from build123d import *

# Parameters (mm, degrees)
SKETCH1_W                                       = 67
SKETCH1_H                                       = 24
BOSS_EXTRUDE1_DEPTH                             = 3.175
CSK_FOR_M2_FLAT_HEAD_MACHINE_SCREW1_D           = 2.2
CSK_FOR_M2_FLAT_HEAD_MACHINE_SCREW1_CSINK_D     = 4.4
CSK_FOR_M2_FLAT_HEAD_MACHINE_SCREW1_CSINK_ANGLE = 90
CHAMFER1_SIZE                                   = 2
CHAMFER1_SIZE2                                  = 2.383507185
SKETCH4_W                                       = 55
SKETCH4_H                                       = 10
CUT_EXTRUDE1_DEPTH                              = 36.725769761
FILLET2_R                                       = 2
FILLET4_R                                       = 3
FILLET5_R                                       = 2


with BuildPart() as part:
    # Sketch1 → Boss-Extrude1 (new body)
    with BuildSketch(Plane(origin=(0, 0, 0), x_dir=(1, 0, 0), z_dir=(0, 1, 0))):
        Rectangle(SKETCH1_W, SKETCH1_H)
    extrude(amount=BOSS_EXTRUDE1_DEPTH)

    # CSK for M2 Flat Head Machine Screw1 (through all)
    with Locations(Plane(origin=(0, 3.175, 0), x_dir=(1, 0, 0), z_dir=(0, 1, 0))):
        with Locations((-30.7, 8.5), (-30.7, -2.5), (30.7, -2.5), (30.7, 8.5)):
            CounterSinkHole(CSK_FOR_M2_FLAT_HEAD_MACHINE_SCREW1_D / 2, CSK_FOR_M2_FLAT_HEAD_MACHINE_SCREW1_CSINK_D / 2, counter_sink_angle=CSK_FOR_M2_FLAT_HEAD_MACHINE_SCREW1_CSINK_ANGLE)

    # Chamfer1
    chamfer1_edges = [part.edges().sort_by_distance(p)[0] for p in [
        (0, 0, 12),
    ]]
    chamfer1_side = [part.faces().sort_by_distance(p)[0] for p in [
        (0, 1.5875, 12),
    ]]
    chamfer(chamfer1_edges, length=CHAMFER1_SIZE, length2=CHAMFER1_SIZE2, reference=chamfer1_side[0])

    # Sketch4 → Cut-Extrude1 (cut, through all)
    with BuildSketch(Plane(origin=(0, 3.175, 0), x_dir=(1, 0, 0), z_dir=(0, 1, 0))):
        with Locations((0, 12)):
            Rectangle(SKETCH4_W, SKETCH4_H)
    extrude(amount=-CUT_EXTRUDE1_DEPTH, mode=Mode.SUBTRACT)

    # Fillet2
    fillet2_edges = [part.edges().sort_by_distance(p)[0] for p in [
        (0, 0, 9.616492815),
    ]]
    fillet(fillet2_edges, radius=FILLET2_R)

    # Fillet4
    fillet4_edges = [part.edges().sort_by_distance(p)[0] for p in [
        (-27.5, 1.5875, -7),
        (27.5, 1.5875, -7),
    ]]
    fillet(fillet4_edges, radius=FILLET4_R)

    # Fillet5
    fillet5_edges = [part.edges().sort_by_distance(p)[0] for p in [
        (33.5, 1.5875, -12),
        (33.5, 2.5875, 12),
        (-33.5, 2.5875, 12),
        (-27.5, 1.5875, -12),
        (27.5, 1.5875, -12),
        (-33.5, 1.5875, -12),
    ]]
    fillet(fillet5_edges, radius=FILLET5_R - 0.0001)  # a hair under: the kernel refuses the full size


solid = part.part
Could you check a few things on this model? Use its own coordinates, in mm. A direction names the side the tool comes from. Coordinates: 2 decimals unless noted, no trailing zeros. Loops run counter-clockwise (first coordinate to the right, second up) from the corner with the lowest first, then second, coordinate; pieces in that order, holes last.
1. Imagine slicing it at B-B (z = -8.5). Please give me the cut outline in (x, y) (3 decimals), and give its area (3 significant figures).
2. For faces 1 (the face through (28.07, 1.57, -11.4)), 2 (the face through (-32.9, 1.61, -11.43)), which set-ups out of +Z, -Z, +X, -X, +Y, -Y let a thin tool reach every point of the face, with its end or its side?
3. We'd pull the mould along Z, two halves only. Please class faces 3 (the face through (-33.5, 2, 0)), 4 (the face through (31.57, 1.02, -7.83)), 5 (the face through (-26.64, 1.57, -7.9)), 6 (the face through (33.15, 2.09, 11.13)): released by +Z, released by -Z, zero draft, split by the parting line, or undercut.
4. Imagine slicing it at C-C (x = 13). Please give me the cut outline in (y, z) (3 decimals).
5. For P1, Ø3, axis at x = -30.7, z = -8.5, coming from the +Y side (3 decimals); P2, Ø8, axis at x = 5, z = 6, coming from the -Y side; P3, Ø1.6, axis at x = 7.5, y = 1, coming from the -Z side, each with a flat end and sliding along its axis, tell me the tip position at first contact or that it passes through.
6. I need wall thicknesses on L1, parallel to Z at x = -30.7, y = 1.25; L2, parallel to X at y = 1.6, z = -8.5; L3, parallel to Z at x = 30.7, y = 1.35. Which ranges of each line are inside material? Lowest first, please.
7. Imagine slicing it at A-A (x = -30.7). Please give me the cut outline in (y, z) (3 decimals).
Computed values:
1. outline: (-33.5, 0) - (-31.8, 0) - (-31.8, 2.075) - (-32.9, 3.175) - (-33.5, 3.175) - close; (-29.6, 0) - (-27.098, 0) - (-27.098, 3.175) - (-28.5, 3.175) - (-29.6, 2.075) - close; (27.098, 0) - (29.6, 0) - (29.6, 2.075) - (28.5, 3.175) - (27.098, 3.175) - close; (31.8, 0) - (33.5, 0) - (33.5, 3.175) - (32.9, 3.175) - (31.8, 2.075) - close
1. area: 24.3 mm2
2. face 1: -Z, +Y, -Y
2. face 2: -Z, -X, +Y, -Y
3. face 3: zero draft
3. face 4: undercut
3. face 5: released by -Z
3. face 6: released by +Z
4. outline: (0, -7) - (3.175, -7) - (3.175, 12) - (2, 12) - (0.468, 10.174) arc R2 ccw to (0, 8.889) - close
5. P1: stops at y = 2.475
5. P2: stops at y = 0
5. P3: stops at z = -7
6. L1: z = -12 to -9.6, -7.4 to 1.4, 3.6 to 11.11
6. L2: x = -33.5 to -31.8, -29.6 to -27.1, 27.1 to 29.6, 31.8 to 33.5
6. L3: z = -12 to -9.6, -7.4 to 1.4, 3.6 to 11.23
7. outline: (0, -12) - (3.175, -12) - (3.175, -10.7) - (2.075, -9.6) - (0, -9.6) - close; (0, -7.4) - (2.075, -7.4) - (3.175, -6.3) - (3.175, 0.3) - (2.075, 1.4) - (0, 1.4) - close; (0, 3.6) - (2.075, 3.6) - (3.175, 4.7) - (3.175, 12) - (2, 12) - (0.468, 10.174) arc R2 ccw to (0, 8.889) - close
